Source: CAD feature listing. Evaluate the final solid. Frame: model axes, mm. A direction names the side the tool comes from. Give positions to 0.01 mm unless a question says otherwise; leave off trailing zeros. Write each loop counter-clockwise with the first axis right and the second up, starting at its lowest first coordinate (ties: lowest second). Pieces come first, ordered by that corner, then holes.
```python
from build123d import *

# Parameters (mm, degrees)
F1_DEPTH = 170
F2_R     = 3
F2_R_2   = 2
F3_DEPTH = 5
F4_DEPTH = 7.501


with BuildPart() as f1:
    # F0 (on Front) → F1 (new body)
    with BuildSketch(Plane.XZ):
        with BuildLine():
            Line((-45.006957, 32.445839), (-55.806957, 32.445839))
            Line((-55.806957, 32.445839), (-55.806957, 31.445839))
            ThreePointArc((-55.806957, 31.445839), (-55.765201, 31.421253), (-55.724493, 31.394966))
            Line((-55.724493, 31.394966), (-55.206957, 31.075689))
            Line((-55.206957, 31.075689), (-55.311685, 30.905929))
            ThreePointArc((-55.311685, 30.905929), (-55.401245, 29.77366), (-56.406957, 29.245839))
            Line((-56.406957, 29.245839), (-56.406957, 24.945839))
            Line((-56.406957, 24.945839), (-44.406957, 24.945839))
            Line((-44.406957, 24.945839), (-44.406957, 29.245839))
            ThreePointArc((-44.406957, 29.245839), (-45.255625, 29.582815), (-45.606948, 30.425645))
            ThreePointArc((-45.606948, 30.425645), (-45.444735, 31.016774), (-45.006957, 31.445839))
            Line((-45.006957, 31.445839), (-45.006957, 32.445839))
        make_face()
        with BuildLine():
            ThreePointArc((-55.724493, 31.394966), (-55.484164, 31.179085), (-55.311685, 30.905929))
            Line((-55.311685, 30.905929), (-55.206957, 31.075689))
            Line((-55.206957, 31.075689), (-55.724493, 31.394966))
        make_face()
    extrude(amount=F1_DEPTH)

    # F2 (on face) → F3 (cut)
    with BuildSketch(Plane.XY.offset(32.445839)):
        with Locations((-50.406957, -160)):
            Circle(F2_R)
        with Locations((-50.406957, -160)):
            Circle(F2_R_2, mode=Mode.SUBTRACT)
        with Locations((-50.406957, -135)):
            Circle(F2_R)
        with Locations((-50.406957, -135)):
            Circle(F2_R_2, mode=Mode.SUBTRACT)
        with Locations((-50.406957, -110)):
            Circle(F2_R)
        with Locations((-50.406957, -110)):
            Circle(F2_R_2, mode=Mode.SUBTRACT)
        with Locations((-50.406957, -85)):
            Circle(F2_R)
        with Locations((-50.406957, -85)):
            Circle(F2_R_2, mode=Mode.SUBTRACT)
        with Locations((-50.406957, -60)):
            Circle(F2_R)
        with Locations((-50.406957, -60)):
            Circle(F2_R_2, mode=Mode.SUBTRACT)
        with Locations((-50.406957, -35)):
            Circle(F2_R)
        with Locations((-50.406957, -35)):
            Circle(F2_R_2, mode=Mode.SUBTRACT)
        with Locations((-50.406957, -10)):
            Circle(F2_R)
        with Locations((-50.406957, -10)):
            Circle(F2_R_2, mode=Mode.SUBTRACT)
    extrude(amount=-F3_DEPTH, mode=Mode.SUBTRACT)

    # F2 (on face) → F4 (cut, through all)
    with BuildSketch(Plane.XY.offset(32.445839)):
        with Locations((-50.406957, -160)):
            Circle(F2_R_2)
        with Locations((-50.406957, -135)):
            Circle(F2_R_2)
        with Locations((-50.406957, -110)):
            Circle(F2_R_2)
        with Locations((-50.406957, -85)):
            Circle(F2_R_2)
        with Locations((-50.406957, -60)):
            Circle(F2_R_2)
        with Locations((-50.406957, -35)):
            Circle(F2_R_2)
        with Locations((-50.406957, -10)):
            Circle(F2_R_2)
    extrude(amount=-F4_DEPTH, mode=Mode.SUBTRACT)


solid = f1.part
```
1. Cut plane C-C, the plane x = -50.25. State how many separate pieces and enclosed holes the cut face has, then the cut area to 3 significant figures.
2. Line query: L1, parallel to X at y = -135, z = 25.9; L2, parallel to Z at x = -49, y = -158.5; L3, parallel to Z at x = -55.5, y = -26.5. Output: solid intervals per line, ascending.
3. Access query for faces 1 (the flat face through (-48, -36, 27.446)), 2 (the cylindrical face through (-50.667, -108.017, 26.213)). Directions: +Z, -Z, +X, -X, +Y, -Y. A direction counts if a zero-diameter tool reaches every point of the face in a straight line with its end or side. Return the directions, or none.
4. Contact query for flat-ended pins moving along their axis: P1, Ø3, axis at x = -49.5, y = -135, coming from the +Z side; P2, Ø3.5, axis at x = -50.41, y = -160, coming from the -Z side; P3, Ø1.1, axis at y = -75, z = 32, coming from the -X side. Output: stop coordinate, or through.
5. Cut plane B-B, the plane y = -40.5. Return the cut outline in (x, z).
6. Cut plane A-A, the plane y = -85. Return the cut outline in (x, z).
Response values:
1. separate pieces: 8
1. enclosed holes: 0
1. area: 996 mm2
2. L1: x = -56.41 to -52.41, -48.41 to -44.41
2. L2: z = 24.95 to 27.45
2. L3: z = 24.95 to 29.64, 31.2 to 32.45
3. face 1: +Z
3. face 2: +Z, -Z
4. P1: stops at z = 27.45
4. P2: passes through
4. P3: stops at x = -55.81
5. outline: (-56.41, 24.95) - (-44.41, 24.95) - (-44.41, 29.25) arc R1.18 cw to (-45.61, 30.43) arc R1.18 cw to (-45.01, 31.45) - (-45.01, 32.45) - (-55.81, 32.45) - (-55.81, 31.45) arc R1.18 cw to (-55.72, 31.39) arc R1.18 cw to (-55.31, 30.91) arc R1.18 cw to (-56.41, 29.25) - close
6. outline: (-56.41, 24.95) - (-52.41, 24.95) - (-52.41, 27.45) - (-53.41, 27.45) - (-53.41, 32.45) - (-55.81, 32.45) - (-55.81, 31.45) arc R1.18 cw to (-55.72, 31.39) arc R1.18 cw to (-55.31, 30.91) arc R1.18 cw to (-56.41, 29.25) - close; (-48.41, 24.95) - (-44.41, 24.95) - (-44.41, 29.25) arc R1.18 cw to (-45.61, 30.43) arc R1.18 cw to (-45.01, 31.45) - (-45.01, 32.45) - (-47.41, 32.45) - (-47.41, 27.45) - (-48.41, 27.45) - close
